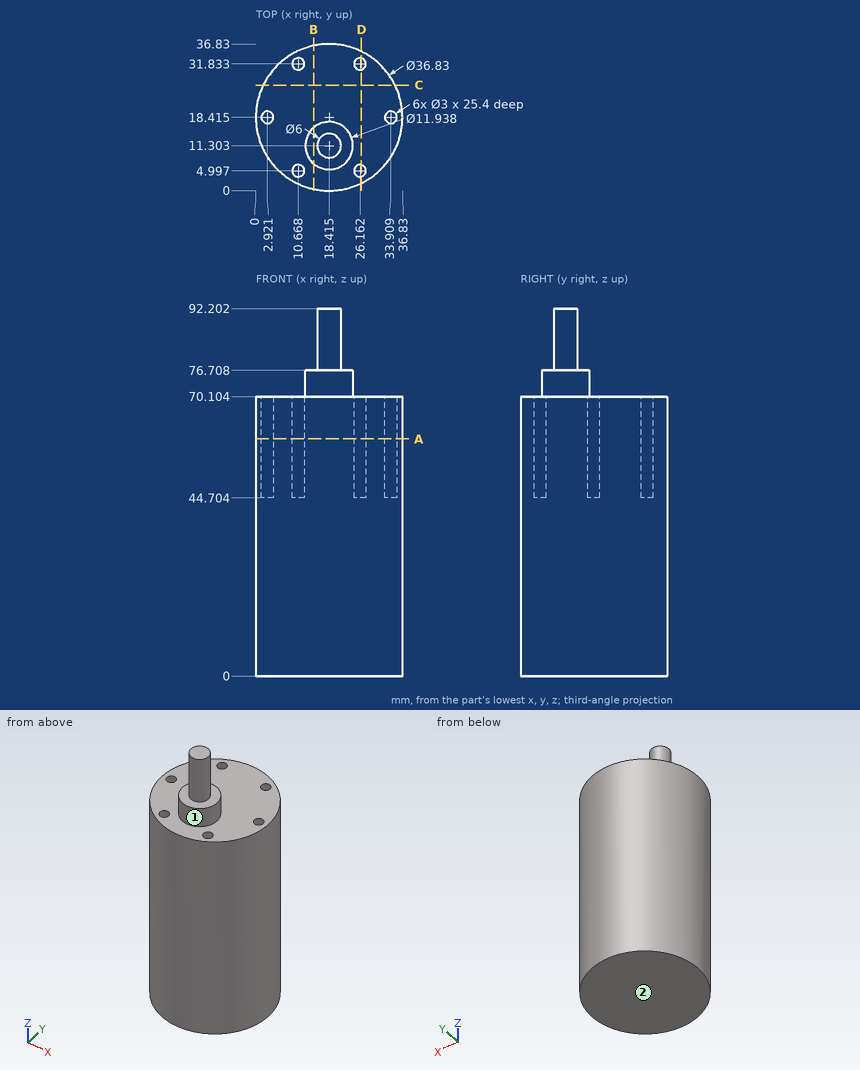
Study the drawing (mm; zero at the part's minimum x, y, z) and answer. A direction names the side the tool comes from. Give positions to 0.01 mm unless a question says otherwise; leave off trailing zeros. Write each loop counter-clockwise with the first axis right and the second up, starting at its lowest first coordinate (ties: lowest second). Pieces come first, ordered by that corner, then holes. Notation, with made-up numbers: (32.5, 86) - (78.5, 86) arc R30 ccw to (78.5, 108) - close; hole circle Ø6 at (-22, 16.5). An arc over 180 degrees is marked (long way). One line per question, with ' | ' between items. Start each with the question number.
1. Section A-A, the plane z = 59.5 is taken. Determine the outline of the cut face in (x, y) (1 decimal).
2. Straight lines are drawn through the part: line 1 (Z direction, x = 5, y = 14); line 2 (Z direction, x = 24, y = 11.5); line 3 (X direction, y = 23.5, z = 51.5). For each, find the intervals that lie inside material, in ascending order.
3. For the marked faces 1 and 2, determine the directions among +Z, -Z, +X, -X, +Y, -Y from which every point of the face is accessible in a straight line to the end or side of a thin tool.
4. Section B-B, the plane x = 14.5 is taken. Determine the outline of the cut face in (y, z).
5. Section D-D, the plane x = 26.5 is taken. Determine the outline of the cut face in (y, z) (1 decimal).
6. Section C-C, the plane y = 26.5 is taken. Determine the outline of the cut face in (x, z).
7. Given P1, Ø6, axis at y = 23, z = 73, coming from the -X side; P2, Ø5, axis at x = 26.16, y = 31.83, coming from the +Z side; P3, Ø8, axis at x = 9.5, z = 39, coming from the -Y side, each flat-ended and moving along its own axis, determine where each tip first touches the part or whether it passes through.
Result:
1) outline: circle Ø36.8 at (18.4, 18.4); hole circle Ø3 at (2.9, 18.4); hole circle Ø3 at (10.7, 5); hole circle Ø3 at (10.7, 31.8); hole circle Ø3 at (26.2, 5); hole circle Ø3 at (26.2, 31.8); hole circle Ø3 at (33.9, 18.4)
2) line 1: z = 0 to 70.1 | line 2: z = 0 to 76.71 | line 3: x = 0.72 to 36.11
3) face 1: +Z | face 2: -Z, +X, -X, +Y, -Y
4) outline: (0.42, 0) - (36.41, 0) - (36.41, 70.1) - (15.81, 70.1) - (15.81, 76.71) - (6.8, 76.71) - (6.8, 70.1) - (0.42, 70.1) - close
5) outline: (1.9, 0) - (35, 0) - (35, 70.1) - (33.3, 70.1) - (33.3, 44.7) - (30.4, 44.7) - (30.4, 70.1) - (6.5, 70.1) - (6.5, 44.7) - (3.5, 44.7) - (3.5, 70.1) - (1.9, 70.1) - close
6) outline: (1.87, 0) - (34.96, 0) - (34.96, 70.1) - (1.87, 70.1) - close
7) P1: stops at x = 0.4 | P2: stops at z = 70.1 | P3: stops at y = 0.67
